The listing builds one solid part. Answer for the finished solid, in the listing's coordinates (mm). Round coordinates to 2 decimals unless told otherwise and drop trailing zeros. Order: outer loops, then holes, each group sorted by start corner. A loop starts at its lowest first (then second) coordinate and runs counter-clockwise, first axis right, second up. Notation, with made-up numbers: (-15, 68) - (21, 68) arc R24 cw to (21, 105) - close; hole circle Ø9 at (76, 0). An arc over 180 degrees is marked (long way). Use CSV: the item, a comma, the result in double quotes. Start each with the question number.
Item 1: Find section D-D, the plane z = -7. Give the vertices of the cut face in (x, y), plus the area to 3 significant figures.
Item 2: Find section A-A, the plane z = 0. Give the vertices of the cut face in (x, y), plus the area to 3 significant figures.
Item 3: A flat-ended cylindrical pin translates along its axis: P1, Ø6, axis at x = -36.63, z = -9.24, coming from the +Y side. Find the tip coordinate at first contact, or state that the pin passes through.
Item 4: Find section B-B, the plane x = -26. Give the vertices of the cut face in (y, z).
Item 5: Straight lines are drawn through the part: line 1 along Z through (x, y) = (25.5, 0.3); line 2 along X through (y, z) = (1.75, 8); line 3 along Z through (x, y) = (38, 1.95). For each, find the intervals that lie inside material, in ascending order. Write a range as [from, to].
Item 6: Find section C-C, the plane z = -20.5. Give the vertices of the cut face in (x, y), plus the area to 3 significant figures.
```python
from build123d import *

# Parameters (mm, degrees)
SKETCH1_W           = 101.6
SKETCH1_H           = 50.8
BOSS_EXTRUDE1_DEPTH = 2.54
CUT_EXTRUDE1_DEPTH  = 57.852894385
CUT_EXTRUDE2_DEPTH  = 57.852894385
SKETCH4_R           = 3.302
CUT_EXTRUDE3_DEPTH  = 57.852894385


with BuildPart() as part:
    # Sketch1 → Boss-Extrude1 (new body)
    with BuildSketch(Plane(origin=(0, 0, 0), x_dir=(1, 0, 0), z_dir=(0, 1, 0))):
        Rectangle(SKETCH1_W, SKETCH1_H)
        with BuildLine():
            Line((-33.02, 15.24), (33.02, 15.24))
            ThreePointArc((33.02, 15.24), (34.544, 13.716), (33.02, 12.192))
            Line((33.02, 12.192), (33.02, -12.192))
            ThreePointArc((33.02, -12.192), (34.544, -13.716), (33.02, -15.24))
            Line((33.02, -15.24), (-33.02, -15.24))
            ThreePointArc((-33.02, -15.24), (-34.544, -13.716), (-33.02, -12.192))
            Line((-33.02, -12.192), (-33.02, 12.192))
            ThreePointArc((-33.02, 12.192), (-34.544, 13.716), (-33.02, 15.24))
        make_face(mode=Mode.SUBTRACT)
    extrude(amount=BOSS_EXTRUDE1_DEPTH)

    # Sketch2 → Cut-Extrude1 (cut, through all)
    with BuildSketch(Plane(origin=(0, 2.54, 0), x_dir=(1, 0, 0), z_dir=(0, 1, 0))):
        with BuildLine():
            Line((-44.759454191, -18.898986355), (-39.679454191, -18.898986355))
            ThreePointArc((-39.679454191, -18.898986355), (-37.139454191, -21.438986355), (-39.679454191, -23.978986355))
            Line((-39.679454191, -23.978986355), (-44.759454191, -23.978986355))
            ThreePointArc((-44.759454191, -23.978986355), (-47.299454191, -21.438986355), (-44.759454191, -18.898986355))
        make_face()
        with BuildLine():
            Line((-28.249454191, -23.978986355), (-23.169454191, -23.978986355))
            ThreePointArc((-23.169454191, -23.978986355), (-20.629454191, -21.438986355), (-23.169454191, -18.898986355))
            Line((-23.169454191, -18.898986355), (-28.249454191, -18.898986355))
            ThreePointArc((-28.249454191, -18.898986355), (-30.789454191, -21.438986355), (-28.249454191, -23.978986355))
        make_face()
        with BuildLine():
            Line((-11.739454191, -23.978986355), (-6.659454191, -23.978986355))
            ThreePointArc((-6.659454191, -23.978986355), (-4.119454191, -21.438986355), (-6.659454191, -18.898986355))
            Line((-6.659454191, -18.898986355), (-11.739454191, -18.898986355))
            ThreePointArc((-11.739454191, -18.898986355), (-14.279454191, -21.438986355), (-11.739454191, -23.978986355))
        make_face()
        with BuildLine():
            Line((4.770545809, -23.978986355), (9.850545809, -23.978986355))
            ThreePointArc((9.850545809, -23.978986355), (12.390545809, -21.438986355), (9.850545809, -18.898986355))
            Line((9.850545809, -18.898986355), (4.770545809, -18.898986355))
            ThreePointArc((4.770545809, -18.898986355), (2.230545809, -21.438986355), (4.770545809, -23.978986355))
        make_face()
        with BuildLine():
            Line((21.280545809, -23.978986355), (26.360545809, -23.978986355))
            ThreePointArc((26.360545809, -23.978986355), (28.900545809, -21.438986355), (26.360545809, -18.898986355))
            Line((26.360545809, -18.898986355), (21.280545809, -18.898986355))
            ThreePointArc((21.280545809, -18.898986355), (18.740545809, -21.438986355), (21.280545809, -23.978986355))
        make_face()
        with BuildLine():
            Line((37.790545809, -23.978986355), (42.870545809, -23.978986355))
            ThreePointArc((42.870545809, -23.978986355), (45.410545809, -21.438986355), (42.870545809, -18.898986355))
            Line((42.870545809, -18.898986355), (37.790545809, -18.898986355))
            ThreePointArc((37.790545809, -18.898986355), (35.250545809, -21.438986355), (37.790545809, -23.978986355))
        make_face()
        with BuildLine():
            Line((-28.249454191, 18.898986355), (-23.169454191, 18.898986355))
            ThreePointArc((-23.169454191, 18.898986355), (-20.629454191, 21.438986355), (-23.169454191, 23.978986355))
            Line((-23.169454191, 23.978986355), (-28.249454191, 23.978986355))
            ThreePointArc((-28.249454191, 23.978986355), (-30.789454191, 21.438986355), (-28.249454191, 18.898986355))
        make_face()
        with BuildLine():
            Line((37.790545809, 18.898986355), (42.870545809, 18.898986355))
            ThreePointArc((42.870545809, 18.898986355), (45.410545809, 21.438986355), (42.870545809, 23.978986355))
            Line((42.870545809, 23.978986355), (37.790545809, 23.978986355))
            ThreePointArc((37.790545809, 23.978986355), (35.250545809, 21.438986355), (37.790545809, 18.898986355))
        make_face()
        with BuildLine():
            Line((21.280545809, 18.898986355), (26.360545809, 18.898986355))
            ThreePointArc((26.360545809, 18.898986355), (28.900545809, 21.438986355), (26.360545809, 23.978986355))
            Line((26.360545809, 23.978986355), (21.280545809, 23.978986355))
            ThreePointArc((21.280545809, 23.978986355), (18.740545809, 21.438986355), (21.280545809, 18.898986355))
        make_face()
        with BuildLine():
            Line((4.770545809, 18.898986355), (9.850545809, 18.898986355))
            ThreePointArc((9.850545809, 18.898986355), (12.390545809, 21.438986355), (9.850545809, 23.978986355))
            Line((9.850545809, 23.978986355), (4.770545809, 23.978986355))
            ThreePointArc((4.770545809, 23.978986355), (2.230545809, 21.438986355), (4.770545809, 18.898986355))
        make_face()
        with BuildLine():
            Line((-11.739454191, 18.898986355), (-6.659454191, 18.898986355))
            ThreePointArc((-6.659454191, 18.898986355), (-4.119454191, 21.438986355), (-6.659454191, 23.978986355))
            Line((-6.659454191, 23.978986355), (-11.739454191, 23.978986355))
            ThreePointArc((-11.739454191, 23.978986355), (-14.279454191, 21.438986355), (-11.739454191, 18.898986355))
        make_face()
        with BuildLine():
            Line((-44.759454191, 18.898986355), (-39.679454191, 18.898986355))
            ThreePointArc((-39.679454191, 18.898986355), (-37.139454191, 21.438986355), (-39.679454191, 23.978986355))
            Line((-39.679454191, 23.978986355), (-44.759454191, 23.978986355))
            ThreePointArc((-44.759454191, 23.978986355), (-47.299454191, 21.438986355), (-44.759454191, 18.898986355))
        make_face()
    extrude(amount=-CUT_EXTRUDE1_DEPTH, mode=Mode.SUBTRACT)

    # Sketch3 → Cut-Extrude2 (cut, through all)
    with BuildSketch(Plane(origin=(0, 2.54, 0), x_dir=(1, 0, 0), z_dir=(0, 1, 0))):
        with BuildLine():
            Line((-33.02, -2.54), (-39.214035088, -2.54))
            ThreePointArc((-39.214035088, -2.54), (-41.754035088, 0), (-39.214035088, 2.54))
            Line((-39.214035088, 2.54), (-33.02, 2.54))
            ThreePointArc((-33.02, 2.54), (-30.48, 0), (-33.02, -2.54))
        make_face()
        with BuildLine():
            Line((33.02, -2.54), (39.214035088, -2.54))
            ThreePointArc((39.214035088, -2.54), (41.754035088, 0), (39.214035088, 2.54))
            Line((39.214035088, 2.54), (33.02, 2.54))
            ThreePointArc((33.02, 2.54), (30.48, 0), (33.02, -2.54))
        make_face()
    extrude(amount=-CUT_EXTRUDE2_DEPTH, mode=Mode.SUBTRACT)

    # Sketch4 → Cut-Extrude3 (cut, through all)
    with BuildSketch(Plane(origin=(0, 2.54, 0), x_dir=(1, 0, 0), z_dir=(0, 1, 0))):
        with Locations(Location((-36.633918246, -7.763735779, 0), (0, 0, 270))):
            Circle(SKETCH4_R)
        with Locations(Location((-36.633918246, 9.236264221, 0), (0, 0, 270))):
            Circle(SKETCH4_R)
        with Locations(Location((38.366081754, -7.763735779, 0), (0, 0, 270))):
            Circle(SKETCH4_R)
        with Locations(Location((38.366081754, 9.236264221, 0), (0, 0, 270))):
            Circle(SKETCH4_R)
    extrude(amount=-CUT_EXTRUDE3_DEPTH, mode=Mode.SUBTRACT)


solid = part.part
```
Worked out:
1,outline,"(-50.8, 0) - (-39.06, 0) - (-39.06, 2.54) - (-50.8, 2.54) - close; (-34.2, 0) - (-33.02, 0) - (-33.02, 2.54) - (-34.2, 2.54) - close; (33.02, 0) - (35.94, 0) - (35.94, 2.54) - (33.02, 2.54) - close; (40.8, 0) - (50.8, 0) - (50.8, 2.54) - (40.8, 2.54) - close"
1,area,"65.6 mm²"
2,outline,"(-50.8, 0) - (-41.75, 0) - (-41.75, 2.54) - (-50.8, 2.54) - close; (41.75, 0) - (50.8, 0) - (50.8, 2.54) - (41.75, 2.54) - close"
2,area,"46.0 mm²"
3,P1,"passes through"
4,outline,"(0, -25.4) - (2.54, -25.4) - (2.54, -23.98) - (0, -23.98) - close; (0, -18.9) - (2.54, -18.9) - (2.54, -15.24) - (0, -15.24) - close; (0, 15.24) - (2.54, 15.24) - (2.54, 18.9) - (0, 18.9) - close; (0, 23.98) - (2.54, 23.98) - (2.54, 25.4) - (0, 25.4) - close"
5,line 1,"z = [-25.4, -23.98], [-18.9, -15.24], [15.24, 18.9], [23.98, 25.4]"
5,line 2,"x = [-50.8, -39.93], [-33.34, -33.02], [33.02, 35.07], [41.66, 50.8]"
5,line 3,"z = [-25.4, -23.98], [-18.9, -12.52], [-5.95, -2.54], [2.54, 4.48], [11.05, 18.9], [23.98, 25.4]"
6,outline,"(-50.8, 0) - (-47.12, 0) - (-47.12, 2.54) - (-50.8, 2.54) - close; (-37.32, 0) - (-30.61, 0) - (-30.61, 2.54) - (-37.32, 2.54) - close; (-20.81, 0) - (-14.1, 0) - (-14.1, 2.54) - (-20.81, 2.54) - close; (-4.3, 0) - (2.41, 0) - (2.41, 2.54) - (-4.3, 2.54) - close; (12.21, 0) - (18.92, 0) - (18.92, 2.54) - (12.21, 2.54) - close; (28.72, 0) - (35.43, 0) - (35.43, 2.54) - (28.72, 2.54) - close; (45.23, 0) - (50.8, 0) - (50.8, 2.54) - (45.23, 2.54) - close"
6,area,"109 mm²"
